Could you check a few things on this model? Use its own coordinates, in mm. Give positions to 0.01 mm unless a question says otherwise; leave off trailing zeros. Write each loop counter-clockwise with the first axis right and the second up, starting at its lowest first coordinate (ties: lowest second). Pieces come first, ordered by that corner, then holes. Notation, with made-up numbers: (27.5, 27.25) - (66.5, 27.25) arc R27 ccw to (66.5, 51.25) - close; hole circle Ø8 at (43, 41). An arc over 180 degrees is marked (long way). Use one line per item in the form item = value.
```python
from build123d import *

# Parameters (mm, degrees)
SKETCH_1_W               = 100
SKETCH_1_H               = 80
SKETCH_1_R               = 30
EXTRUDE_1_DEPTH          = 3
SKETCH_2_R               = 2.1
CUT_EXTRUDE_1_DEPTH      = 10
PATTERN_CIRCULAR_1_COUNT = 4


with BuildPart() as part:
    # 草图1 → 凸台-拉伸1 (new body)
    with BuildSketch(Plane(origin=(0, 0, 0), x_dir=(1, 0, 0), z_dir=(0, 1, 0))):
        Rectangle(SKETCH_1_W, SKETCH_1_H)
        Circle(SKETCH_1_R, mode=Mode.SUBTRACT)
    extrude(amount=EXTRUDE_1_DEPTH)

    # 草图2 → 切除-拉伸1 (cut)
    with BuildSketch(Plane(origin=(0, 3, 0), x_dir=(1, 0, 0), z_dir=(0, 1, 0))):
        with Locations((27, 27)):
            Circle(SKETCH_2_R)
    cut_extrude_1 = extrude(amount=-CUT_EXTRUDE_1_DEPTH, mode=Mode.SUBTRACT)

    # 阵列(圆周)1: 切除-拉伸1 ×4 about axis
    pattern_circular_1_axis = Axis((0, 0, 0), (0, 1, 0))
    for i in range(1, PATTERN_CIRCULAR_1_COUNT):
        add(cut_extrude_1.rotate(pattern_circular_1_axis, i * 360 / PATTERN_CIRCULAR_1_COUNT), mode=Mode.SUBTRACT)


solid = part.part
```
1. Imagine slicing it at A-A, the plane x = 18. List the corners of the cut face in (y, z) for me, and give its area (3 significant figures).
Response values:
outline = (0, -40) - (3, -40) - (3, -24) - (0, -24) - close; (0, 24) - (3, 24) - (3, 40) - (0, 40) - close
area = 96.0 mm²
2. If we mould it in two halves opening along X, with no side actions, what happens to faces 1 (the face through (-25.137, 1.521, -27.969)), 2 (the face through (-34, 3, -1)), 3 (the face through (50, 1, 1))? For each: pulls with the +X half, pulls with the -X half, needs draft (parallel to the pull), parting line crosses it, or undercut.
Response values:
face_1 = undercut
face_2 = needs draft
face_3 = pulls with the +X half
3. If I drill on line 1 (X direction, y = 1.3, z = 0); line 2 (X direction, y = 0.75, z = -27); line 3 (Z direction, x = 27, y = 2.35), over which ranges is the centre line in solid material (lowest first)? Write a range as from..to.
Response values:
line_1 = -50..-30, 30..50
line_2 = -50..-29.1, -24.9..-13.08, 13.08..24.9, 29.1..50
line_3 = -40..-29.1, -24.9..-13.08, 13.08..24.9, 29.1..40
4. Imagine slicing it at C-C, the plane y = 1.2. List the corners of the cut face in (x, z) for me, and give its area (3 significant figures).
Response values:
outline = (-50, -40) - (50, -40) - (50, 40) - (-50, 40) - close; hole circle Ø60 at (0, 0); hole circle Ø4.2 at (-27, -27); hole circle Ø4.2 at (-27, 27); hole circle Ø4.2 at (27, -27); hole circle Ø4.2 at (27, 27)
area = 5,120 mm²
5. Imagine slicing it at D-D, the plane z = 10.5. List the corners of the cut face in (x, y) for me.
Response values:
outline = (-50, 0) - (-28.1, 0) - (-28.1, 3) - (-50, 3) - close; (28.1, 0) - (50, 0) - (50, 3) - (28.1, 3) - close
6. Imagine slicing it at B-B, the plane z = 27. List the corners of the cut face in (x, y) for me, and give its area (3 significant figures).
Response values:
outline = (-50, 0) - (-29.1, 0) - (-29.1, 3) - (-50, 3) - close; (-24.9, 0) - (-13.08, 0) - (-13.08, 3) - (-24.9, 3) - close; (13.08, 0) - (24.9, 0) - (24.9, 3) - (13.08, 3) - close; (29.1, 0) - (50, 0) - (50, 3) - (29.1, 3) - close
area = 196 mm²
7. For pin 1 (4 mm diameter, centred on x = -27, z = 27, fed in from +Y), with a flat end and sliding along its axis, tell me the tip position at first contact or that it passes through.
Response values:
pin_1 = through
